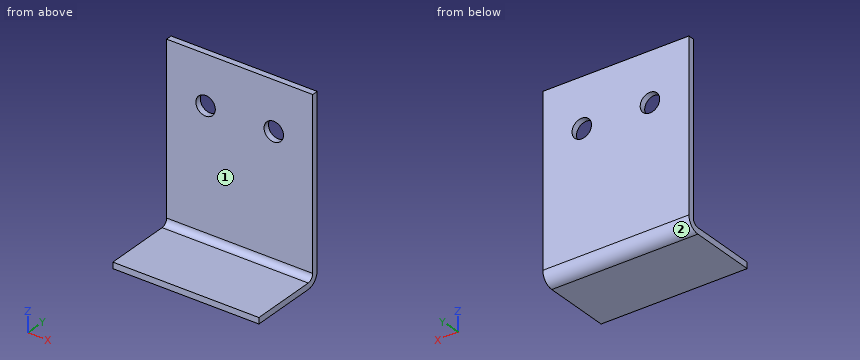
```python
from build123d import *

# Parameters (mm, degrees)
SKETCH1_W                    = 38.1
SKETCH1_H                    = 46.99
BOSS_EXTRUDE1_DEPTH          = 1.5875
EDGE_FLANGE1_STRIP_W         = 9.525
EDGE_FLANGE1_STRIP_H         = 1.5875
EDGE_FLANGE1_STRIP_CUT_DEPTH = 38.1
EDGE_FLANGE1_DEPTH           = 38.1
SKETCH13_R                   = 2.54
CUT_EXTRUDE1_DEPTH           = 25.4


# Sheet-metal steps are written as plain solids
with BuildPart() as part:
    # Sketch1 → Boss-Extrude1 (new body)
    with BuildSketch(Plane(origin=(0, 0, 0), x_dir=(1, 0, 0), z_dir=(0, 1, 0))):
        Rectangle(SKETCH1_W, SKETCH1_H)
    extrude(amount=BOSS_EXTRUDE1_DEPTH)

    # Edge-Flange1 strip (across the edge) → Edge-Flange1 strip cut (cut)
    with BuildSketch(Plane(origin=(-19.05, 0, -23.495), x_dir=(0, 0, 1), z_dir=(1, 0, 0))):
        with Locations((-1.5875, -0.79375)):
            Rectangle(EDGE_FLANGE1_STRIP_W, EDGE_FLANGE1_STRIP_H)
    extrude(amount=EDGE_FLANGE1_STRIP_CUT_DEPTH, mode=Mode.SUBTRACT)

    # Edge-Flange1 section (across the edge) → Edge-Flange1 (add)
    with BuildSketch(Plane(origin=(-19.05, 0, -23.495), x_dir=(0, 0, 1), z_dir=(1, 0, 0))):
        with BuildLine():
            Line((0, 1.5875), (0, 19.05))
            Line((0, 19.05), (1.5875, 19.05))
            Line((1.5875, 19.05), (1.5875, 1.5875))
            ThreePointArc((1.5875, 1.5875), (2.052467985, 0.464967985), (3.175, 0))
            Line((3.175, 0), (3.175, -1.5875))
            ThreePointArc((3.175, -1.5875), (0.92993597, -0.65756403), (0, 1.5875))
        make_face()
    extrude(amount=EDGE_FLANGE1_DEPTH)

    # Sketch13 → Cut-Extrude1 (cut)
    with BuildSketch(Plane(origin=(0, 1.5875, 0), x_dir=(1, 0, 0), z_dir=(0, 1, 0))):
        with Locations(Location((8.89, -10.795, 0), (0, 0, 270))):
            Circle(SKETCH13_R)
        with Locations(Location((-8.89, -10.795, 0), (0, 0, 270))):
            Circle(SKETCH13_R)
    extrude(amount=-CUT_EXTRUDE1_DEPTH, mode=Mode.SUBTRACT)


solid = part.part
```
Can you work these out from the model? Positions are in its coordinate system, mm. Face numbers are marked on the shaded views. A direction names the side the tool comes from. Round coordinates to 2 decimals unless told otherwise and drop trailing zeros. Answer in a Markdown table with one row per item.
Item 1: Will these pins go through, and if not, where does the flat tip stop? P1, Ø8.5, axis at x = -1.5, y = -10, coming from the +Z side; P2, Ø3, axis at x = -4, z = -5, coming from the -Y side.
Answer block:
| item | result |
|---|---|
| P1 | z = -21.91 |
| P2 | y = 0 |
Item 2: On a 3-axis mill with a long thin cutter (end or side, diameter ignored), from which of +Z, -Z, +X, -X, +Y, -Y can I reach the whole of each face in a straight line? I mean the marked faces 1 and 2. Say none if no direction works.
Answer block:
| item | result |
|---|---|
| face 1 | +Z, +X, -X, -Y |
| face 2 | -Z, +X, -X, +Y |
Item 3: If I drill on probe 1 along Y at (x, z) = (-17, 9); probe 2 along Z at (x, y) = (-10.5, -14.25) (1 decimal); probe 3 along Z at (x, y) = (10, -0.5), over which ranges is the centre line in solid material (lowest first)?
Answer block:
| item | result |
|---|---|
| probe 1 | 0 to 1.59 |
| probe 2 | -23.5 to -21.9 |
| probe 3 | -23.3 to -21.48 |
